```python
from build123d import *

# Parameters (mm, degrees)
SKETCH2_W          = 0.25
SKETCH2_H          = 3
CUT_EXTRUDE1_DEPTH = 0.25


with BuildPart() as part:
    # Sketch1 → Revolve1 (revolve)
    with BuildSketch(Plane(origin=(0, 0, 0), x_dir=(0, 0, -1), z_dir=(1, 0, 0)), mode=Mode.PRIVATE) as revolve1_sk:
        with BuildLine():
            Line((0, 10), (0, 15))
            Line((0, 15), (2.324948115, 15))
            ThreePointArc((2.324948115, 15), (2.468342225, 14.954788011), (2.559871271, 14.835505036))
            Line((2.559871271, 14.835505036), (4.623950135, 9.164494964))
            ThreePointArc((4.623950135, 9.164494964), (4.715479181, 9.045211989), (4.85887329, 9))
            Line((4.85887329, 9), (25.5, 9))
            ThreePointArc((25.5, 9), (25.853553391, 8.853553391), (26, 8.5))
            Line((26, 8.5), (26, 0))
            Line((26, 0), (23.5, 0))
            Line((23.5, 0), (23.5, 3))
            Line((23.5, 3), (2.5, 3))
            Line((2.5, 3), (2.5, 10))
            Line((2.5, 10), (0, 10))
        make_face()
    revolve(revolve1_sk.sketch.rotate(Axis((0, 0, 0), (0, 0, -1)), 90), axis=Axis((0, 0, 0), (0, 0, -1)))

    # Sketch2 → Cut-Extrude1 (cut)
    with BuildSketch(Plane(origin=(0, 0, -26), x_dir=(-1, 0, 0), z_dir=(0, 0, -1))):
        with Locations((0, 8)):
            Rectangle(SKETCH2_W, SKETCH2_H)
    extrude(amount=-CUT_EXTRUDE1_DEPTH, mode=Mode.SUBTRACT)


solid = part.part
```
For this review, take the finished solid that the model builds, in its own axes (mm). A direction names the side the tool comes from. Round coordinates to 2 decimals unless told otherwise and drop trailing zeros. Order: outer loops, then holes, each group sorted by start corner. A loop starts at its lowest first (then second) coordinate and runs counter-clockwise, first axis right, second up.
Q1. We need section C-C, the plane z = -3.5. Give the boundary of the cut face in (x, y), plus the area to 3 significant figures.
Findings below:
outline: circle Ø24.51 at (0, 0); hole circle Ø6 at (0, 0)
area: 443 mm2
Q2. Machinability: for faces 5 (the cylindrical face through (-10, 0, -1)), 6 (the flat face through (-3, 10, 0)), which of the approach directions +Z, -Z, +X, -X, +Y, -Y give a long, thin tool a straight path to every point of the face, cutting with its end or side? Answer none if there is none.
Findings below:
face 5: +Z
face 6: +Z, +X, -X, +Y, -Y
Q3. Mouldability with a two-part tool opening along X and no side actions: class faces 1 (the flat face through (0, 0, -23.5)), 2 (the flat face through (-2.1, -2.4, -2.5)), 3 (the cylindrical face through (-6.633, -6.083, -15.324)), 4 (the flat face through (0, 0, -26)) as pulls with the +X half, pulls with the -X half, needs draft (parallel to the pull), parting line crosses it, or undercut.
Findings below:
face 1: undercut
face 2: undercut
face 3: parting line crosses it
face 4: needs draft
Q4. We need section B-B, the plane z = -6.5. Give the boundary of the cut face in (x, y), plus the area to 3 significant figures.
Findings below:
outline: circle Ø18 at (0, 0); hole circle Ø6 at (0, 0)
area: 226 mm2
Q5. We need section A-A, the plane y = 0. Give the boundary of the cut face in (x, z).
Findings below:
outline: (-15, -2.32) arc R0.25 ccw to (-14.84, -2.56) - (-9.16, -4.62) arc R0.25 cw to (-9, -4.86) - (-9, -25.5) arc R0.5 ccw to (-8.5, -26) - (8.5, -26) arc R0.5 ccw to (9, -25.5) - (9, -4.86) arc R0.25 cw to (9.16, -4.62) - (14.84, -2.56) arc R0.25 ccw to (15, -2.32) - (15, 0) - (10, 0) - (10, -2.5) - (3, -2.5) - (3, -23.5) - (-3, -23.5) - (-3, -2.5) - (-10, -2.5) - (-10, 0) - (-15, 0) - close
Q6. Wall thickness on line 1 (Y direction, x = 0, z = -1.75); line 2 (Y direction, x = 0, z = -9.5); line 3 (Z direction, x = -2.5, y = 0): over which ranges is each line inside the solid? List them lowest first.
Findings below:
line 1: y = -15 to -10, 10 to 15
line 2: y = -9 to -3, 3 to 9
line 3: z = -26 to -23.5
Q7. Insertion check: P1, Ø1.5, axis at x = -2.5, y = -8, coming from the +Z side; P2, Ø5.5, axis at x = 0, y = 0, coming from the +Z side; P3, Ø3, axis at x = -3.5, z = -7.5, coming from the -Y side. Each pin has a flat end and moves straight along its axis. Give the tip position at first contact, or say it passes through.
Findings below:
P1: stops at z = -2.5
P2: stops at z = -23.5
P3: stops at y = -8.77
